Input: part model. Units: mm. Frame: model coordinates. Face numbers are marked on the shaded views. A direction names the side the tool comes from. Round coordinates to 2 decimals unless told otherwise and drop trailing zeros. Loops run counter-clockwise (first coordinate to the right, second up) from the corner with the lowest first, then second, coordinate; pieces in that order, holes last. Notation, with made-up numbers: (56, 77.5) - (65, 77.5) arc R26 cw to (65, 91.5) - close; hole circle Ø2 at (-11.75, 17.25). An arc over 180 degrees is marked (long way). Write each question's results on one line, items separated by ' | '.
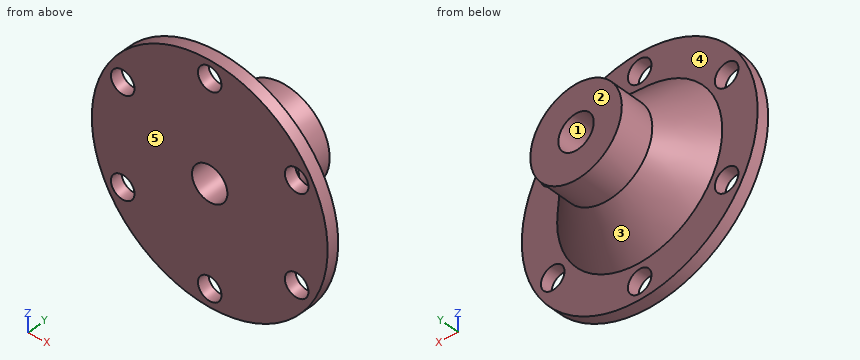
from build123d import *

# Parameters (mm, degrees)
SKETCH1_R           = 127
BOSS_EXTRUDE1_DEPTH = 12.7
SKETCH2_R           = 12.7
CUT_EXTRUDE1_DEPTH  = 12.7
SKETCH3_R           = 88.9
BOSS_EXTRUDE2_DEPTH = 39.6875
CHAMFER1_SIZE       = 39.6875
SKETCH4_R           = 19.05
CUT_EXTRUDE5_DEPTH  = 88.4555
BOSS_EXTRUDE3_START = 36.5125
SKETCH5_R           = 49.276
SKETCH5_R_2         = 19.05
BOSS_EXTRUDE3_DEPTH = 36.5125


with BuildPart() as part:
    # Sketch1 → Boss-Extrude1 (new body)
    with BuildSketch(Plane(origin=(0, 0, 0), x_dir=(1, 0, 0), z_dir=(0, 1, 0))):
        with Locations(Location((0, 0, 0), (0, 0, 270))):
            Circle(SKETCH1_R)
    extrude(amount=BOSS_EXTRUDE1_DEPTH)

    # Sketch2 → Cut-Extrude1 (cut)
    with BuildSketch(Plane(origin=(0, 12.7, 0), x_dir=(1, 0, 0), z_dir=(0, 1, 0))):
        with Locations(Location((0, 107.95, 0), (0, 0, 270))):
            Circle(SKETCH2_R)
        with Locations(Location((0, -107.95, 0), (0, 0, 270))):
            Circle(SKETCH2_R)
        with Locations(Location((-93.6625, -53.975, 0), (0, 0, 270))):
            Circle(SKETCH2_R)
        with Locations(Location((-93.6625, 53.975, 0), (0, 0, 270))):
            Circle(SKETCH2_R)
        with Locations(Location((93.6625, 53.975, 0), (0, 0, 270))):
            Circle(SKETCH2_R)
        with Locations(Location((93.6625, -53.975, 0), (0, 0, 270))):
            Circle(SKETCH2_R)
    extrude(amount=-CUT_EXTRUDE1_DEPTH, mode=Mode.SUBTRACT)

    # Sketch3 → Boss-Extrude2 (add)
    with BuildSketch(Plane(origin=(0, 12.7, 0), x_dir=(1, 0, 0), z_dir=(0, 1, 0))):
        with Locations(Location((0, 0, 0), (0, 0, 90))):
            Circle(SKETCH3_R)
    extrude(amount=BOSS_EXTRUDE2_DEPTH)

    # Chamfer1
    chamfer1_edges = [part.edges().sort_by_distance(p)[0] for p in [
        (0, 52.3875, 88.9),
    ]]
    chamfer(chamfer1_edges, length=CHAMFER1_SIZE - 0.0001)  # a hair under: the kernel refuses the full size

    # Sketch4 → Cut-Extrude5 (cut)
    with BuildSketch(Plane(origin=(0, 52.3875, 0), x_dir=(1, 0, 0), z_dir=(0, 1, 0))):
        with Locations(Location((0, 0, 0), (0, 0, 270))):
            Circle(SKETCH4_R)
    extrude(amount=-CUT_EXTRUDE5_DEPTH, mode=Mode.SUBTRACT)

    # Sketch5 → Boss-Extrude3 (add)
    with BuildSketch(Plane(origin=(0, 52.3875, 0), x_dir=(1, 0, 0), z_dir=(0, 1, 0)).offset(BOSS_EXTRUDE3_START)):
        with Locations(Location((0, 0, 0), (0, 0, 270))):
            Circle(SKETCH5_R)
        with Locations(Location((0, 0, 0), (0, 0, 270))):
            Circle(SKETCH5_R_2, mode=Mode.SUBTRACT)
    extrude(amount=-BOSS_EXTRUDE3_DEPTH)


solid = part.part
1. Section query D-D, the plane y = 58. Output: boundary loops of the cut face in (x, z).
Answer:
outline: circle Ø98.55 at (0, 0); hole circle Ø38.1 at (0, 0)
2. Section query B-B, the plane x = 99. Output: boundary loops of the cut face in (y, z), plus the area to 3 significant figures.
Answer:
outline: (0, -79.55) - (12.7, -79.55) - (12.7, -65.5) - (0, -65.5) - close; (0, -42.45) - (12.7, -42.45) - (12.7, 42.45) - (0, 42.45) - close; (0, 65.5) - (12.7, 65.5) - (12.7, 79.55) - (0, 79.55) - close | area: 1,440 mm^2
3. Section query C-C, the plane x = 0. Count the separate pieces of the cut face and the enclosed holes in it, plus the area to 3 significant figures.
Answer:
separate pieces: 4 | enclosed holes: 0 | area: 8,270 mm^2
4. Set-up query: the marked faces 4 and 5. Return all of +Z, -Z, +X, -X, +Y, -Y with unobstructed straight access to the full face (end or side cutting, diameter ignored); none if empty.
Answer:
face 4: +Y | face 5: +Z, -Z, +X, -X, -Y
5. Contact query for flat-ended pins moving along their axis: pin 1 (6 mm diameter, centred on x = -10.5, z = 88, fed in from -Y); pin 2 (20.5 mm diameter, centred on x = 0, z = -107.95, fed in from -Y); pin 3 (12 mm diameter, centred on y = 53, z = 18.5, fed in from -X); pin 4 (4 mm diameter, centred on x = 2.5, y = 59.5, fed in from -Z). Output: stop coordinate, or through.
Answer:
pin 1: y = 0 | pin 2: through | pin 3: x = -51.69 | pin 4: z = -49.27
6. Mould query, pull axis X, two halves, no side actions, for the marked faces 1, 2 and 3. Classes: pulls with the +X half, pulls with the -X half, needs draft (parallel to the pull), parting line crosses it, or undercut.
Answer:
face 1: undercut | face 2: needs draft | face 3: parting line crosses it
7. Line query: line 1 (Y direction, x = -6.5, z = 90); line 2 (Z direction, x = -5, y = 79); line 3 (X direction, y = 7.5, z = 107.95). Output: solid intervals per line, ascending. Write a range as [from, to].
Answer:
line 1: [0, 12.7] | line 2: [-49.02, -18.38], [18.38, 49.02] | line 3: [-66.9, -12.7], [12.7, 66.9]
